The model under review builds one solid part; all positions refer to its coordinate system, in mm. Round coordinates to 2 decimals unless told otherwise and drop trailing zeros. Loops run counter-clockwise (first coordinate to the right, second up) from the corner with the lowest first, then second, coordinate; pieces in that order, holes last. Notation, with made-up numbers: (-36.5, -22) -> (-17.5, -22) arc R24 ccw to (-17.5, -7) -> close; hole circle Ø11 at (57.5, 60.5). An arc over 180 degrees is marked (long way). Use a Markdown table: item, result. Add a question column.
1) Consider section B-B on x = 4.5. Give the boundary of the cut face in (y, z).
2) Wall thickness on probe 1 along Z at (x, y) = (19.5, 5.5); probe 2 along Z at (x, y) = (20.5, 8.75): over which ranges is each line inside the solid? List them lowest first.
3) Consider section A-A on z = 161.5. Give the boundary of the cut face in (x, y).
4) Consider section D-D on x = 41.5. Give the boundary of the cut face in (y, z), plus the area to 3 significant figures.
5) Consider section C-C on y = 1.5. Give the boundary of the cut face in (x, z).
from build123d import *

# Parameters (mm, degrees)
ESQUISSE1_W        = 44
ESQUISSE1_H        = 22
BOSS_EXTRU_1_DEPTH = 137
BOSS_EXTRU_2_DEPTH = 44
ESQUISSE3_R        = 2.5
BOSS_EXTRU_3_DEPTH = 173


with BuildPart() as part:
    # Esquisse1 → Boss.-Extru.1 (new body)
    with BuildSketch(Plane.XY):
        with Locations((22, 11)):
            Rectangle(ESQUISSE1_W, ESQUISSE1_H)
    extrude(amount=BOSS_EXTRU_1_DEPTH)

    # Esquisse2 → Boss.-Extru.2 (add)
    with BuildSketch(Plane(origin=(44, 0, 0), x_dir=(0, 0, -1), z_dir=(1, 0, 0))):
        with BuildLine():
            Line((-137, 22), (-137, 0))
            ThreePointArc((-137, 0), (-147, 11), (-137, 22))
        make_face()
    extrude(amount=-BOSS_EXTRU_2_DEPTH)

    # Esquisse3 → Boss.-Extru.3 (add)
    with BuildSketch(Plane(origin=(0, 0, 0), x_dir=(-1, 0, 0), z_dir=(0, 0, -1))):
        with Locations((-41.5, 14)):
            Circle(ESQUISSE3_R)
        with Locations((-41.5, 8)):
            Circle(ESQUISSE3_R)
    extrude(amount=-BOSS_EXTRU_3_DEPTH)


solid = part.part
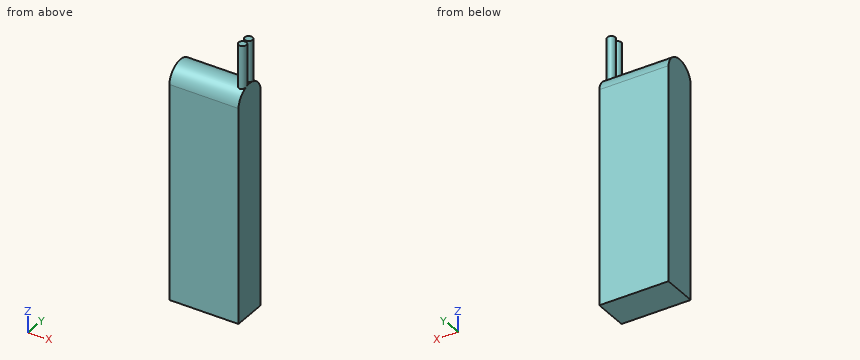
Result set:
| question | item | result |
|---|---|---|
| 1 | outline | (0, 0) -> (22, 0) -> (22, 137) arc R11.05 ccw to (0, 137) -> close |
| 2 | probe 1 | 0 to 145.53 |
| 2 | probe 2 | 0 to 146.77 |
| 3 | outline | circle Ø5 at (41.5, 8); circle Ø5 at (41.5, 14) |
| 4 | outline | (0, 0) -> (22, 0) -> (22, 137) arc R11.05 ccw to (16.5, 145.53) -> (16.5, 173) -> (11.5, 173) -> (11.5, 146.99) arc R11.05 ccw to (10.5, 146.99) -> (10.5, 173) -> (5.5, 173) -> (5.5, 145.53) arc R11.05 ccw to (0, 137) -> close |
| 4 | area | 3,450 mm2 |
| 5 | outline | (0, 0) -> (44, 0) -> (44, 141.59) -> (0, 141.59) -> close |
